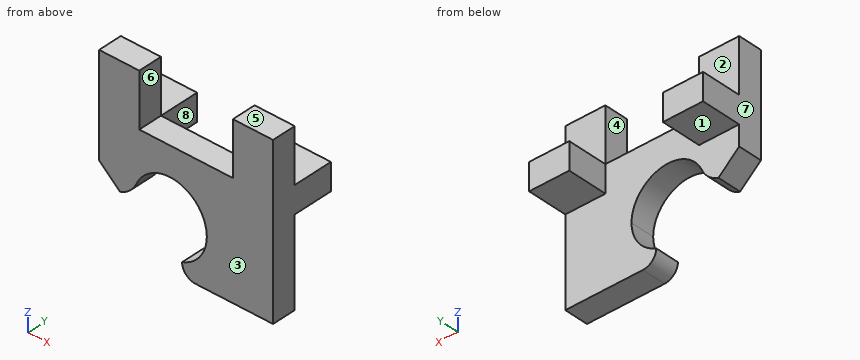
```python
from build123d import *

# Parameters (mm, degrees)
BOSS_EXTRUDE1_DEPTH = 1.8
FILLET1_R           = 2
FILLET3_R           = 1
SKETCH2_W           = 3
SKETCH2_H           = 2
BOSS_EXTRUDE2_DEPTH = 3


# Some blends are built 0.0001 mm under size
with BuildPart() as part:
    # Sketch1 → Boss-Extrude1 (new body)
    with BuildSketch(Plane(origin=(0, 0, 0), x_dir=(1, 0, 0), z_dir=(0, 1, 0))):
        with BuildLine():
            Line((6.5, 2.5), (6.5, 0))
            Line((6.5, 0), (6.5, -4))
            Line((6.5, -4), (3.5, -4))
            Line((3.5, -4), (3.5, 0))
            Line((3.5, 0), (-3.5, 0))
            Line((-3.5, 0), (-3.5, -4))
            Line((-3.5, -4), (-6.5, -4))
            Line((-6.5, -4), (-6.5, 0))
            Line((-6.5, 0), (-6.5, 2.5))
            Line((-6.5, 2.5), (-6.5, 3.5))
            Line((-6.5, 3.5), (-4.95, 4.9))
            Line((-4.95, 4.9), (-3.95, 4.9))
            ThreePointArc((-3.95, 4.9), (-1.2, 2.15), (1.55, 4.9))
            ThreePointArc((1.55, 4.9), (1.040256682, 6.494913791), (-0.3, 7.498557292))
            Line((-0.3, 7.498557292), (-0.3, 8.498557292))
            Line((-0.3, 8.498557292), (6.5, 8.498557292))
            Line((6.5, 8.498557292), (6.5, 4.9))
            Line((6.5, 4.9), (6.5, 2.5))
        make_face()
    extrude(amount=BOSS_EXTRUDE1_DEPTH)

    # Fillet1
    # the kernel refuses this fillet: 2 mm, written as the material it takes off along each edge
    with BuildSketch(Plane(origin=(-3.95, -2.821440468, -4.9), x_dir=(0.20519567041703113, 0, 0.9787209698591858), z_dir=(0, 1, 0))) as fillet1_piece_1:
        with BuildLine():
            CenterArc((1.538967528, -1.95744194), FILLET1_R, 101.840953646, 48.860489585)
            Line((-0.20519567, -0.97872097), (-0.240078934, -0.95914655))
            ThreePointArc((-0.240078934, -0.95914655), (-0.141746674, -0.481152658), (-0.039148839, 0.008207827))
            Line((-0.039148839, 0.008207827), (0.008207827, 0.039148839))
            ThreePointArc((0.008207827, 0.039148839), (0.564288094, -0.018517333), (1.12036836, 0.039148839))
            Line((1.12036836, 0.039148839), (1.128576187, 0))
        make_face()
    extrude(amount=7.442880936, mode=Mode.SUBTRACT)

    # Fillet3
    fillet3_edges = [part.edges().sort_by_distance(p)[0] for p in [
        (-0.3, 0.9, -8.498557292),
    ]]
    fillet(fillet3_edges, radius=FILLET3_R - 0.0001)  # a hair under: the kernel refuses the full size

    # Sketch2 → Boss-Extrude2 (add)
    with BuildSketch(Plane.XZ):
        with Locations((5, -1)):
            Rectangle(SKETCH2_W, SKETCH2_H)
        with Locations((-5, -1)):
            Rectangle(SKETCH2_W, SKETCH2_H)
    extrude(amount=BOSS_EXTRUDE2_DEPTH)


with BuildPart() as body_2:
    # Mirror3: mirrored copy
    add(part.part.mirror(Plane(origin=(0, 0, 0), x_dir=(0, 0, 1), z_dir=(0, -1, 0))))


solid = body_2.part
```
Model file for the job. Use its own axes, mm. Face numbers are marked on the shaded views. A direction names the side the tool comes from. Coordinates: 2 decimals unless noted, no trailing zeros. Order: outer loops, then holes, each group sorted by start corner. A loop starts at its lowest first (then second) coordinate and runs counter-clockwise, first axis right, second up. Notation, with made-up numbers: (45.5, 81.25) - (65.5, 81.25) arc R31 cw to (65.5, 109.25) - close; hole circle Ø9 at (30.5, -9). An arc over 180 degrees is marked (long way). Return JSON: item names as keys, results as strings. Group by question number.
1) Saw through at B-B, the plane z = 0.75. Write the cut outline in (x, y), plus the area to 3 significant figures.
2) Tool access for the marked faces 1, 2, 3 and 4: list every direction of +Z, -Z, +X, -X, +Y, -Y with a clear straight run to the whole face (end or side of a thin tool).
3) Mould opens along X. For the marked faces 5, 6, 7 and 8 say: released by +X, released by -X, zero draft, split by the parting line, or undercut.
4) Saw through at A-A, the plane y = 1.6. Write the cut outline in (x, z).
5) Saw through at C-C, the plane x = 3.75. Write the cut outline in (y, z).
6) Probe line 1 (X direction, y = -0.2, z = 1.25); line 2 (Y direction, x = 3, z = -6); line 3 (Z direction, x = -4.25, y = 1.3). List the from-to ranges inside material, lowest first. Write a range as from..to.
7) Flat gauge pins, fed straight in: P1, Ø1.5, axis at x = -5, y = 2, coming from the +Z side; P2, Ø7, axis at x = -1, z = -6, coming from the +Y side; P3, Ø1.5, axis at x = 5.5, y = 1, coming from the -Z side. Where does each tip first touch, or does it go through?
Values found:
{
 "1": {"outline": "(-6.5, -1.8) - (-3.5, -1.8) - (-3.5, 0) - (-6.5, 0) - close; (3.5, -1.8) - (6.5, -1.8) - (6.5, 0) - (3.5, 0) - close", "area": "10.8 mm²"},
 "2": {"face 1": "-Z, +X, -X, +Y", "face 2": "+Z, +X, -X, +Y", "face 3": "+Z, -Z, +X, -X, -Y", "face 4": "+Z, +Y, -Y"},
 "3": {"face 5": "zero draft", "face 6": "undercut", "face 7": "released by -X", "face 8": "undercut"},
 "4": {"outline": "(-6.5, -2) - (-3.5, -2) - (-3.5, 0) - (-6.5, 0) - close; (3.5, -2) - (6.5, -2) - (6.5, 0) - (3.5, 0) - close"},
 "5": {"outline": "(-1.8, -8.5) - (0, -8.5) - (0, -2) - (3, -2) - (3, 0) - (0, 0) - (0, 4) - (-1.8, 4) - close"},
 "6": {"line 1": "x = -6.5..-3.5, 3.5..6.5", "line 2": "y = -1.8..0", "line 3": "z = -2..0"},
 "7": {"P1": "stops at z = 0", "P2": "stops at y = 0", "P3": "stops at z = -2"}
}
